from build123d import *

# Parameters (mm, degrees)
F1_DEPTH      = 6
F3_DEPTH      = 2
F6_DEPTH      = 3.2
F7_R          = 1.75
F8_DEPTH      = 4.2
F8_DEPTH_BACK = 0.8


with BuildPart() as f1:
    # F0 (on Front) → F1 (new body)
    with BuildSketch(Plane.XZ):
        with BuildLine():
            Line((15, 0), (13, 0))
            ThreePointArc((13, 0), (12.6330653649, -0.0697532727), (12.3173205132, -0.2692820528))
            Line((12.3173205132, -0.2692820528), (8.3653589736, -3.9614358943))
            ThreePointArc((8.3653589736, -3.9614358943), (7, -4.5), (5.6346410264, -3.9614358943))
            Line((5.6346410264, -3.9614358943), (1.6826794868, -0.2692820528))
            ThreePointArc((1.6826794868, -0.2692820528), (1.3669346351, -0.0697532727), (1, 0))
            Line((1, 0), (0, 0))
            Line((0, 0), (0, -2))
            Line((0, -2), (0.6055512755, -2))
            Line((0.6055512755, -2), (4.2692820528, -5.4228717887))
            ThreePointArc((4.2692820528, -5.4228717887), (7, -6.5), (9.7307179472, -5.4228717887))
            Line((9.7307179472, -5.4228717887), (13.3944487245, -2))
            Line((13.3944487245, -2), (15, -2))
            Line((15, -2), (15, 0))
        make_face()
    extrude(amount=F1_DEPTH)



with BuildPart() as f1b:
    # F0 (on Front) → F1, piece 2 (new body)
    with BuildSketch(Plane.XZ):
        with BuildLine():
            Line((0, 4.5), (0, 2.5))
            Line((0, 2.5), (1, 2.5))
            Line((1, 2.5), (13, 2.5))
            Line((13, 2.5), (15, 2.5))
            Line((15, 2.5), (15, 3.5))
            ThreePointArc((15, 3.5), (14.7071067812, 4.2071067812), (14, 4.5))
            Line((14, 4.5), (12, 4.5))
            Line((12, 4.5), (12, 7.5))
            Line((12, 7.5), (2, 7.5))
            Line((2, 7.5), (2, 4.5))
            Line((2, 4.5), (0, 4.5))
        make_face()
    extrude(amount=F1_DEPTH)


with BuildPart() as f1_1:
    add(f1.part)

    add(f1b.part)  # F3 merges F1b
    # F2 (on Front) → F3 (join)
    with BuildSketch(Plane.XZ):
        with BuildLine():
            Line((13.3944487245, -2), (15, -2))
            Line((15, -2), (15, 3.5))
            ThreePointArc((15, 3.5), (14.7071067812, 4.2071067812), (14, 4.5))
            Line((14, 4.5), (12, 4.5))
            Line((12, 4.5), (12, 7.5))
            Line((12, 7.5), (2, 7.5))
            Line((2, 7.5), (2, 4.5))
            Line((2, 4.5), (0, 4.5))
            Line((0, 4.5), (0, -2))
            Line((0, -2), (0.6055512755, -2))
            Line((0.6055512755, -2), (4.2692820528, -5.4228717887))
            ThreePointArc((4.2692820528, -5.4228717887), (7, -6.5), (9.7307179472, -5.4228717887))
            Line((9.7307179472, -5.4228717887), (13.3944487245, -2))
        make_face()
    extrude(amount=-F3_DEPTH)

    # F5 (on offset) → F6 (cut)
    with BuildSketch(Plane(origin=(0, 0, 3.3), x_dir=(1, 0, 0), z_dir=(0, 0, -1))):
        Polygon((7, -0.9259818305), (10.4, 1.0370090848), (10.4, 4.9629909152), (10.4, 11.3659846154), (3.6, 11.3659846154), (3.6, 4.9629909152), (3.6, 1.0370090848), align=None)
    extrude(amount=-F6_DEPTH, mode=Mode.SUBTRACT)

    # F7 (on face) → F8 (cut, two sides)
    with BuildSketch(Plane.XY.offset(3.3)) as f8_sk:
        with Locations((7, -3)):
            Circle(F7_R)
    extrude(amount=F8_DEPTH, mode=Mode.SUBTRACT)
    extrude(f8_sk.sketch, amount=-F8_DEPTH_BACK, mode=Mode.SUBTRACT)

    # F9: F1 across plane


with BuildPart() as f1_2:
    add(f1_1.part)
    add(f1_1.part.mirror(Plane.YZ))


solid = f1_2.part
Work out the finished part from the listing and answer in its coordinate system (mm). A direction names the side the tool comes from. Coordinates: 2 decimals unless noted, no trailing zeros. Write each loop counter-clockwise with the first axis right and the second up, starting at its lowest first coordinate (ties: lowest second). Pieces come first, ordered by that corner, then holes.
1. Consider line 1 along X through (y, z) = (-3, 6.95); line 2 along Y through (x, z) = (-7, 7.2); line 3 along Z through (x, y) = (-6, -5.5). Determine where each line is inside the solid, lowest interval first.
Results list:
line 1: x = -12 to -8.75, -5.25 to -2, 2 to 5.25, 8.75 to 12
line 2: y = -6 to -4.75, -1.25 to 2
line 3: z = -6.37 to -4.23, 2.5 to 3.3, 6.5 to 7.5
2. For a pull along Z with two mould halves and no side action, classify faces 1 (the flat face through (8.676, -0.042, 4.878)), 2 (the flat face through (15, -1, -1)), 3 (the flat face through (-13, -2, 4.5)), 4 (the flat face through (-14, -2, -2)) as +Z half, -Z half, draft (parallel to the pull), parting line (faces both ways), or undercut.
Results list:
face 1: undercut
face 2: draft
face 3: +Z half
face 4: -Z half
3. The part is cut by section D-D, the plane y = -3. State how many separate pieces and enclosed holes the cut face has, and give its area (3 significant figures).
Results list:
separate pieces: 4
enclosed holes: 0
area: 137 mm2
4. The part is cut by section C-C, the plane y = 1.5. Write down the section's boundary in (x, z).
Results list:
outline: (-15, -2) - (-13.39, -2) - (-9.73, -5.42) arc R4 ccw to (-4.27, -5.42) - (-0.61, -2) - (0.61, -2) - (4.27, -5.42) arc R4 ccw to (9.73, -5.42) - (13.39, -2) - (15, -2) - (15, 3.5) arc R1 ccw to (14, 4.5) - (12, 4.5) - (12, 7.5) - (2, 7.5) - (2, 4.5) - (-2, 4.5) - (-2, 7.5) - (-12, 7.5) - (-12, 4.5) - (-14, 4.5) arc R1 ccw to (-15, 3.5) - close
5. The part is cut by section B-B, the plane x = 6. Write down the section's boundary in (y, z).
Results list:
outline: (-6, -6.37) - (2, -6.37) - (2, 7.5) - (-1.56, 7.5) - (-1.56, 6.5) - (0.35, 6.5) - (0.35, 3.3) - (-1.56, 3.3) - (-1.56, 2.5) - (0, 2.5) - (0, -4.23) - (-6, -4.23) - close; (-6, 2.5) - (-4.44, 2.5) - (-4.44, 3.3) - (-6, 3.3) - close; (-6, 6.5) - (-4.44, 6.5) - (-4.44, 7.5) - (-6, 7.5) - close
6. For faces 5 (the flat face through (0, -3, 0)), 6 (the flat face through (12, -2, 6)), 7 (the flat face through (0, 0, 1)), 8 (the cylindrical face through (7.81, -4.55, 2.91)), determine the directions among +Z, -Z, +X, -X, +Y, -Y from which every point of the face is accessible in a straight line to the end or side of a thin tool.
Results list:
face 5: +X, -X, -Y
face 6: +Z, +X, +Y, -Y
face 7: -Y
face 8: +Z
7. Flat-ended cylindrical pins translate along their axes: pin 1 (3 mm diameter, centred on x = 3, y = -3, fed in from -Z); pin 2 (2.5 mm diameter, centred on y = -4.5, z = 5.5, fed in from -X); pin 3 (3 mm diameter, centred on x = 1.5, y = -4.5, fed in from -Z). Find the tip coordinate at first contact, or state that the pin passes through.
Results list:
pin 1: stops at z = -5.62
pin 2: stops at x = -14.66
pin 3: stops at z = -4.24
8. The part is cut by section A-A, the plane z = 5.25. Write down the section's boundary in (x, y).
Results list:
outline: (-12, -6) - (-10.4, -6) - (-10.4, -1.04) - (-7, 0.93) - (-3.6, -1.04) - (-3.6, -6) - (-2, -6) - (-2, 2) - (-12, 2) - close; (2, -6) - (3.6, -6) - (3.6, -1.04) - (7, 0.93) - (10.4, -1.04) - (10.4, -6) - (12, -6) - (12, 2) - (2, 2) - close
